Here's how the part is built. I have some questions about the finished solid (model axes, mm). A direction names the side the tool comes from. Round coordinates to 2 decimals unless told otherwise and drop trailing zeros. Write each loop counter-clockwise with the first axis right and the second up, starting at its lowest first coordinate (ties: lowest second). Pieces come first, ordered by that corner, then holes. Notation, with made-up numbers: (14, 35.5) - (20, 35.5) arc R20 ccw to (20, 58.5) - close; hole circle Ø10 at (17, 71). An arc over 180 degrees is marked (long way). Use one line per item in the form item = value. Start each with the question number.
1. We'd pull the mould along Y, two halves only. Please class faces 1 (the cylindrical face through (149.181, 5.634, 2.93)), 2 (the flat face through (152.4, 12, -1)), 3 (the cylindrical face through (-149.269, 5.634, 2.93)), 4 (the flat face through (-2, -19.05, -52)): +Y half, -Y half, draft (parallel to the pull), parting line (faces both ways), or undercut.
2. I want a section at A-A, the plane z = 0. List the corners of the cut face in (x, y) for me.
3. I want a section at B-B, the plane y = 0. List the corners of the cut face in (x, z) for me, plus the area to 3 significant figures.
4. I want a section at D-D, the plane z = -15.5. List the corners of the cut face in (x, y) for me, plus the area to 3 significant figures.
5. Which directions (+Z, -Z, +X, -X, +Y, -Y) give clear straight access to the entire face, cutting with the end or side of a thin tool? Please do faces 5 (the flat face through (-152.4, 12, -1)), 6 (the flat face through (-2, -19.05, 52)), 7 (the cylindrical face through (-2.04, -52.38, 0.88)).
6. Will these pins go through, and if not, where does the flat tip stop? pin 1 (10 mm diameter, centred on x = 28.5, z = 6, fed in from +Y); pin 2 (7.5 mm diameter, centred on x = -50, z = -53, fed in from +Y); pin 3 (4 mm diameter, centred on x = -62.5, z = -22, fed in from +Y); pin 4 (20.5 mm diameter, centred on y = 0, z = 0, fed in from -X).
7. If I drill on line 1 along Y through (x, z) = (149, 0); line 2 along X through (y, z) = (3.5, -32); line 3 along Y through (x, z) = (115, 26.5), over which ranges is the centre line in solid material (lowest first)?
8. I want a section at C-C, the plane y = -42.5. List the corners of the cut face in (x, z) for me, plus the area to 3 significant figures.
```python
from build123d import *

# Parameters (mm, degrees)
SKETCH1_R               = 58.7375
SKETCH1_R_2             = 6.35
BOSS_EXTRUDE1_DEPTH     = 152.4
CUT_EXTRUDE1_DEPTH      = 174.568279972
CUT_EXTRUDE1_DEPTH_BACK = 174.568279972
SKETCH2_W               = 292.1
SKETCH2_H               = 77.7875
SHELL1_START            = -146.05
SHELL1_DEPTH            = 292.1


# Read off the part's stored shape, not the designer's step: Shell1
with BuildPart() as part:
    # Sketch1 → Boss-Extrude1 (new, symmetric)
    with BuildSketch(Plane(origin=(0, 0, 0), x_dir=(0, 0, -1), z_dir=(1, 0, 0))):
        with Locations(Location((0, 0, 0), (0, 0, 180))):
            Circle(SKETCH1_R)
        with Locations(Location((0, 0, 0), (0, 0, 180))):
            Circle(SKETCH1_R_2, mode=Mode.SUBTRACT)
    extrude(amount=BOSS_EXTRUDE1_DEPTH, both=True)

    # Sketch2 → Cut-Extrude1 (cut, two sides: drawn at the far end of the back side and taken through both)
    with BuildSketch(Plane.XY.offset(-CUT_EXTRUDE1_DEPTH_BACK)):
        with Locations((0, 19.84375)):
            Rectangle(SKETCH2_W, SKETCH2_H)
    extrude(amount=CUT_EXTRUDE1_DEPTH + CUT_EXTRUDE1_DEPTH_BACK, mode=Mode.SUBTRACT)

    # Shell1 outline → Shell1 (cut)
    with BuildSketch(Plane.YZ.offset(SHELL1_START)):
        with BuildLine():
            ThreePointArc((-19.05, 48.801103023), (-52.3875, 0), (-19.05, -48.801103023))
            Line((-19.05, -48.801103023), (-19.05, 48.801103023))
        make_face()
    extrude(amount=SHELL1_DEPTH, mode=Mode.SUBTRACT)


solid = part.part
```
Model answer:
q1.face_1 = undercut
q1.face_2 = draft
q1.face_3 = undercut
q1.face_4 = +Y half
q2.outline = (-152.4, -58.74) - (152.4, -58.74) - (152.4, -6.35) - (146.05, -6.35) - (146.05, -52.39) - (-146.05, -52.39) - (-146.05, -6.35) - (-152.4, -6.35) - close; (-152.4, 6.35) - (-146.05, 6.35) - (-146.05, 58.74) - (-152.4, 58.74) - close; (146.05, 6.35) - (152.4, 6.35) - (152.4, 58.74) - (146.05, 58.74) - close
q3.outline = (-152.4, -58.74) - (-146.05, -58.74) - (-146.05, -6.35) - (-152.4, -6.35) - close; (-152.4, 6.35) - (-146.05, 6.35) - (-146.05, 58.74) - (-152.4, 58.74) - close; (146.05, -58.74) - (152.4, -58.74) - (152.4, -6.35) - (146.05, -6.35) - close; (146.05, 6.35) - (152.4, 6.35) - (152.4, 58.74) - (146.05, 58.74) - close
q3.area = 1,330 mm2
q4.outline = (-152.4, -56.66) - (152.4, -56.66) - (152.4, 56.66) - (146.05, 56.66) - (146.05, -50.04) - (-146.05, -50.04) - (-146.05, 56.66) - (-152.4, 56.66) - close
q4.area = 3,370 mm2
q5.face_5 = +Z, -Z, -X, +Y, -Y
q5.face_6 = +Z, -Z, +Y
q5.face_7 = +Y
q6.pin_1 = -51.22
q6.pin_2 = -19.05
q6.pin_3 = -46.57
q6.pin_4 = -152.4
q7.line_1 = -58.74 to -6.35, 6.35 to 58.74
q7.line_2 = -152.4 to -146.05, 146.05 to 152.4
q7.line_3 = -52.42 to -45.19
q8.outline = (-152.4, -40.54) - (152.4, -40.54) - (152.4, 40.54) - (-152.4, 40.54) - close; hole (-146.05, -30.63) - (146.05, -30.63) - (146.05, 30.63) - (-146.05, 30.63) - close
q8.area = 6,820 mm2
